```python
from build123d import *

# Parameters (mm, degrees)
SKETCH1_W           = 25
SKETCH1_H           = 25
BOSS_EXTRUDE1_DEPTH = 4
SKETCH2_R           = 10
CUT_EXTRUDE1_DEPTH  = 3
SKETCH3_R           = 1.25
BOSS_EXTRUDE2_DEPTH = 2
FILLET1_R           = 1
SKETCH4_R           = 1
BOSS_EXTRUDE3_DEPTH = 2


with BuildPart() as part:
    # Sketch1 → Boss-Extrude1 (new body)
    with BuildSketch(Plane(origin=(0, 0, 0), x_dir=(1, 0, 0), z_dir=(0, 1, 0))):
        Rectangle(SKETCH1_W, SKETCH1_H)
    extrude(amount=BOSS_EXTRUDE1_DEPTH)

    # Sketch2 → Cut-Extrude1 (cut)
    with BuildSketch(Plane(origin=(0, 4, 0), x_dir=(1, 0, 0), z_dir=(0, 1, 0))):
        Circle(SKETCH2_R)
    extrude(amount=-CUT_EXTRUDE1_DEPTH, mode=Mode.SUBTRACT)

    # Sketch3 → Boss-Extrude2 (add)
    with BuildSketch(Plane(origin=(0, 1, 0), x_dir=(1, 0, 0), z_dir=(0, 1, 0))):
        Circle(SKETCH3_R)
    extrude(amount=BOSS_EXTRUDE2_DEPTH)

    # Fillet1
    fillet1_edges = [part.edges().sort_by_distance(p)[0] for p in [
        (-1.25, 3, 0),
    ]]
    fillet(fillet1_edges, radius=FILLET1_R)

    # Sketch4 → Boss-Extrude3 (add)
    with BuildSketch(Plane(origin=(0, 4, 0), x_dir=(1, 0, 0), z_dir=(0, 1, 0))):
        with Locations((-10.5, 10.5)):
            Circle(SKETCH4_R)
        with Locations((10.5, 10.5)):
            Circle(SKETCH4_R)
        with Locations((10.5, -10.5)):
            Circle(SKETCH4_R)
        with Locations((-10.5, -10.5)):
            Circle(SKETCH4_R)
    extrude(amount=BOSS_EXTRUDE3_DEPTH)


solid = part.part
```
Geometry: final body of the model. Coordinates: model frame, mm. A direction names the side the tool comes from. Round coordinates to 2 decimals unless told otherwise and drop trailing zeros. Loops run counter-clockwise (first coordinate to the right, second up) from the corner with the lowest first, then second, coordinate; pieces in that order, holes last. Notation, with made-up numbers: (-26, -17) -> (-8, -17) arc R20 ccw to (-8, -6) -> close; hole circle Ø8 at (61.5, 86). An arc over 180 degrees is marked (long way). Use one line per item in the form item = value. Start each with the question number.
1) Section C-C on y = 5.3. Output: boundary loops of the cut face in (x, z), then the cut area to 3 significant figures.
2) Line query: L1, parallel to Z at x = 0, y = 1.75; L2, parallel to Z at x = 0, y = 3.1. Output: solid intervals per line, ascending.
3) Section B-B on x = -10.5. Output: boundary loops of the cut face in (y, z).
4) Draft query along Z for faces 1 (the flat face through (0, 2, 12.5)), 2 (the flat face through (0, 0, 0)), 3 (the cylindrical face through (-2.17, 2.52, 9.76)). Return one class per face: released by +Z, released by -Z, zero draft, split by the parting line, or undercut.
5) Access query for faces 4 (the cylindrical face through (-11.237, 4.986, -11.176)), 5 (the flat face through (-11, 6, 10)). Directions: +Z, -Z, +X, -X, +Y, -Y. A direction counts if a zero-diameter tool reaches every point of the face in a straight line with its end or side. Return the directions, or none.
6) First-contact query: P1, Ø4, axis at x = 5, z = -6.5, coming from the +Y side; P2, Ø1, axis at x = -5, z = 4, coming from the +Y side; P3, Ø1.5, axis at x = -3, z = -1.5, coming from the -Y side. Flat tips, straight axial feed; report the tip coordinate or a pass-through.
7) Section D-D on x = -4.25. Output: boundary loops of the cut face in (y, z).
8) Section A-A on z = 10.5. Output: boundary loops of the cut face in (x, y).
Response:
q1.outline = circle Ø2 at (-10.5, -10.5); circle Ø2 at (-10.5, 10.5); circle Ø2 at (10.5, -10.5); circle Ø2 at (10.5, 10.5)
q1.area = 12.6 mm^2
q2.L1 = -12.5 to -10, -1.25 to 1.25, 10 to 12.5
q2.L2 = -12.5 to -10, 10 to 12.5
q3.outline = (0, -12.5) -> (4, -12.5) -> (4, -11.5) -> (6, -11.5) -> (6, -9.5) -> (4, -9.5) -> (4, 9.5) -> (6, 9.5) -> (6, 11.5) -> (4, 11.5) -> (4, 12.5) -> (0, 12.5) -> close
q4.face_1 = released by +Z
q4.face_2 = zero draft
q4.face_3 = undercut
q5.face_4 = +Y
q5.face_5 = +Z, -Z, +X, -X, +Y
q6.P1 = 4
q6.P2 = 1
q6.P3 = 0
q7.outline = (0, -12.5) -> (4, -12.5) -> (4, -9.05) -> (1, -9.05) -> (1, 9.05) -> (4, 9.05) -> (4, 12.5) -> (0, 12.5) -> close
q8.outline = (-12.5, 0) -> (12.5, 0) -> (12.5, 4) -> (11.5, 4) -> (11.5, 6) -> (9.5, 6) -> (9.5, 4) -> (-9.5, 4) -> (-9.5, 6) -> (-11.5, 6) -> (-11.5, 4) -> (-12.5, 4) -> close
